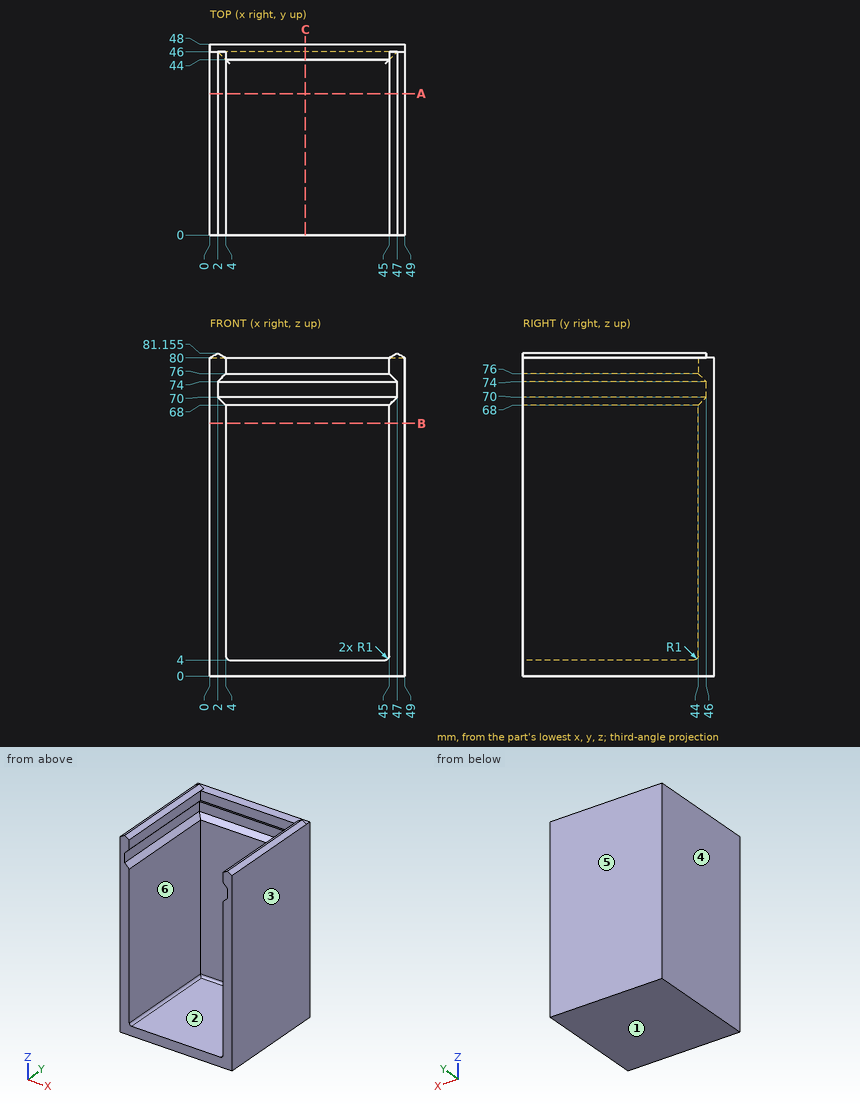
Source: three-view drawing plus pictorial views. Frame: mm from the lowest corner of the part. A direction names the side the tool comes from. Give positions to 0.01 mm unless a question says otherwise; leave off trailing zeros. Write each loop counter-clockwise with the first axis right and the second up, starting at its lowest first coordinate (ties: lowest second). Pieces come first, ordered by that corner, then holes.
(1) Cut plane A-A, the plane y = 35.5. Return loops of the section in (x, z) (1 decimal).
(2) Cut plane B-B, the plane z = 63.5. Return loops of the section in (x, y), then the cut area to 3 significant figures.
(3) Ray query, line 1 (X direction, y = 41, z = 60); line 2 (Z direction, x = 15, y = 16.5); line 3 (Y direction, x = 35, z = 31). Return the intervals inside material, ascending.
(4) Access query for the marked faces 5 and 6. Directions: +Z, -Z, +X, -X, +Y, -Y. A direction counts if a zero-diameter tool reaches every point of the face in a straight line with its end or side. Return the directions, or none.
(5) Mould query, pull axis X, two halves, no side actions, for the marked faces 1, 2, 3 and 4. Classes: released by +X, released by -X, zero draft, split by the parting line, or undercut.
(6) Cut plane C-C, the plane x = 24. Return loops of the section in (y, z).
(7) First-contact query: P1, Ø2, axis at x = 33, y = 46.5, coming from the +Z side; P2, Ø3, axis at x = 33, z = 78, coming from the -Y side; P3, Ø0.6, axis at x = 2, z = 80.5, coming from the +Y side. Flat tips, straight axial feed; report the tip coordinate or a pass-through.
Values follow:
1. outline: (0, 0) - (49, 0) - (49, 80) - (47, 81.2) - (45, 80) - (45, 76) - (47, 74) - (47, 70) - (45, 68) - (45, 5) arc R1 cw to (44, 4) - (5, 4) arc R1 cw to (4, 5) - (4, 68) - (2, 70) - (2, 74) - (4, 76) - (4, 80) - (2, 81.2) - (0, 80) - close
2. outline: (0, 0) - (4, 0) - (4, 44) - (45, 44) - (45, 0) - (49, 0) - (49, 48) - (0, 48) - close
2. area: 548 mm2
3. line 1: x = 0 to 4, 45 to 49
3. line 2: z = 0 to 4
3. line 3: y = 44 to 48
4. face 5: +Z, -Z, +X, -X, +Y
4. face 6: +Z, -Y
5. face 1: zero draft
5. face 2: undercut
5. face 3: released by +X
5. face 4: released by -X
6. outline: (0, 0) - (48, 0) - (48, 80) - (44, 80) - (44, 76) - (46, 74) - (46, 70) - (44, 68) - (44, 5) arc R1 cw to (43, 4) - (0, 4) - close
7. P1: stops at z = 80
7. P2: stops at y = 44
7. P3: stops at y = 46
